The model under review builds one solid part; all positions refer to its coordinate system, in mm. A direction names the side the tool comes from. Round coordinates to 2 decimals unless told otherwise and drop trailing zeros. Write each loop counter-clockwise with the first axis right and the second up, starting at its lowest first coordinate (ties: lowest second). Pieces come first, ordered by that corner, then holes. Notation, with made-up numbers: (-29, -24.5) -> (-23, -24.5) arc R19 ccw to (-23, -15.5) -> close; hole circle Ø11 at (-1, 89). An arc over 180 degrees is marked (long way). Answer in a Markdown table with one row per item. Add a question column.
```python
from build123d import *

# Parameters (mm, degrees)
F3_D           = 13.208
F3_CBORE_D     = 44.45
F3_CBORE_DEPTH = 3.683
F2_W           = 44.336462139
F2_H           = 1.016
F4_DEPTH       = 38.1
F5_SIZE        = 5.08
F6_W           = 101.6
F6_H           = 1
F7_DEPTH       = 0.5


with BuildPart() as f1:
    # F0 (on Front) → F1 (revolve)
    with BuildSketch(Plane.XZ):
        Polygon((-38.227, 0), (0, 0), (0, 25.4), (-44.45, 25.4), (-44.45, 15.875), (-38.227, 15.875), align=None)
    revolve(axis=Axis((0, 0, 19.0648827702), (0, 0, 1)))

    # F3 (through all)
    with Locations(Plane.XY.offset(25.4)):
        with Locations((0, 0)):
            CounterBoreHole(F3_D / 2, F3_CBORE_D / 2, F3_CBORE_DEPTH)

    # F2 (on face) → F4 (cut)
    with BuildSketch(Plane.XY.offset(25.4)):
        with Locations((22.1682310695, -0.508)):
            Rectangle(F2_W, F2_H)
        with BuildLine():
            Line((44.336462139, 0), (44.336462139, -1.016))
            Line((44.336462139, -1.016), (44.4383870544, -1.016))
            ThreePointArc((44.4383870544, -1.016), (44.4470966688, -0.5080331831), (44.45, 0))
            Line((44.45, 0), (44.336462139, 0))
        make_face()
        with BuildLine():
            ThreePointArc((44.45, 0), (44.4470966688, -0.5080331831), (44.4383870544, -1.016))
            Line((44.4383870544, -1.016), (50.8, -1.016))
            Line((50.8, -1.016), (50.8, 0))
            Line((50.8, 0), (44.45, 0))
        make_face()
    extrude(amount=-F4_DEPTH, mode=Mode.SUBTRACT)

    # F5
    f5_edges = [f1.edges().sort_by_distance(p)[0] for p in [
        (-0.508045, -38.223624, 0),
    ]]
    chamfer(f5_edges, length=F5_SIZE)

    # F6 (on face) → F7 (cut)
    with BuildSketch(Plane.XY.offset(25.4)):
        with Locations((0, -25.3804288805)):
            Rectangle(F6_W, F6_H)
        with Locations((0, -30.9059806168)):
            Rectangle(F6_W, F6_H)
        with Locations((2.5503417128, -36.5805682886)):
            Rectangle(F6_W, F6_H)
        with Locations((0.3315322974, 44.9394750249)):
            Rectangle(F6_W, F6_H)
        with Locations((0.3083095216, 40.7329852533)):
            Rectangle(F6_W, F6_H)
        with Locations((0.3083095216, 35.207433517)):
            Rectangle(F6_W, F6_H)
        with Locations((0.6398418191, 29.3503458452)):
            Rectangle(F6_W, F6_H)
        with Locations((0.6398418191, 23.8247941089)):
            Rectangle(F6_W, F6_H)
        with Locations((0.5792960728, 18.6377671853)):
            Rectangle(F6_W, F6_H)
        with Locations((0.5792960728, 13.112215449)):
            Rectangle(F6_W, F6_H)
        with Locations((0.9108283703, 7.2551277772)):
            Rectangle(F6_W, F6_H)
        with Locations((0.9108283703, 1.7295760409)):
            Rectangle(F6_W, F6_H)
        with Locations((0.8876055945, -2.4769137307)):
            Rectangle(F6_W, F6_H)
        with Locations((0.8876055945, -8.0024654671)):
            Rectangle(F6_W, F6_H)
        with Locations((1.2191378919, -13.8595531388)):
            Rectangle(F6_W, F6_H)
        with Locations((1.2191378919, -19.3851048752)):
            Rectangle(F6_W, F6_H)
        with Locations((1.0724808089, -41.2088056254)):
            Rectangle(F6_W, F6_H)
    extrude(amount=-F7_DEPTH, mode=Mode.SUBTRACT)


solid = f1.part
```
1. For L1, parallel to Y at x = 0, z = 23.55 (3 decimals); L2, parallel to Y at x = -7.5, z = 22.25; L3, parallel to Z at x = -17, y = 35 (3 decimals), list the stretches that pass through material, from the lowest coordinate up.
2. Tool access review of faces 1 (the flat face through (26, 0, 13)), 2 (the flat face through (27, 16, 25.4)), 3 (the flat face through (20, 33, 15.875)): name each direction out of +Z, -Z, +X, -X, +Y, -Y from which nothing blocks a thin tool from reaching the whole face with its end or side.
3. Insertion check: pin 1 Ø4 at (x, z) = (16.5, 10.5) entering from -Y; pin 2 Ø2 at (y, z) = (-1.5, 6.5) entering from -X; pin 3 Ø7.5 at (x, z) = (24.5, 17.5) entering from +Y. Each pin has a flat end and moves straight along its axis. Give the tip position at first contact, or say it passes through.
4. Mouldability with a two-part tool opening along X and no side actions: class faces 4 (the flat face through (0, 42, 25.4)), 5 (the flat face through (-5, -5, 21.717)) as pulls with the +X half, pulls with the -X half, needs draft (parallel to the pull), parting line crosses it, or undercut.
5. Add section A-A on z = 7.75. Write out the cut boundary in (x, y).
6. Add section B-B on z = 2.75. Write out the cut boundary in (x, y).
Filled in:
| question | item | result |
|---|---|---|
| 1 | L1 | -44.45 to -22.225, 22.225 to 44.45 |
| 1 | L2 | -43.81 to -20.92, 20.92 to 43.81 |
| 1 | L3 | 15.875 to 24.9 |
| 2 | face 1 | +Z, -Z, +X |
| 2 | face 2 | +Z, +X, -X, +Y, -Y |
| 2 | face 3 | -Z |
| 3 | pin 1 | y = -35.37 |
| 3 | pin 2 | x = -38.22 |
| 3 | pin 3 | y = 39.31 |
| 4 | face 4 | needs draft |
| 4 | face 5 | undercut |
| 5 | outline | (6.53, -1.02) arc R6.6 cw (long way) to (6.6, 0) -> (38.23, 0) arc R38.23 ccw (long way) to (38.21, -1.02) -> close |
| 6 | outline | (6.53, -1.02) arc R6.6 cw (long way) to (6.6, 0) -> (35.9, 0) arc R35.9 ccw (long way) to (35.88, -1.02) -> close |
